Verification items for this drawing (mm, ordinates from the low corner). Give positions to 0.01 mm unless a question says otherwise; leave off trailing zeros. Order: outer loops, then holes, each group sorted by start corner. A loop starts at its lowest first (then second) coordinate and runs counter-clockwise, first axis right, second up. Notation, with made-up numbers: (11.25, -29) -> (33.25, -29) arc R17 ccw to (33.25, -13) -> close; hole circle Ø10 at (84.25, -29). An arc over 180 degrees is marked (long way). One line per question, with ' | ' between items.
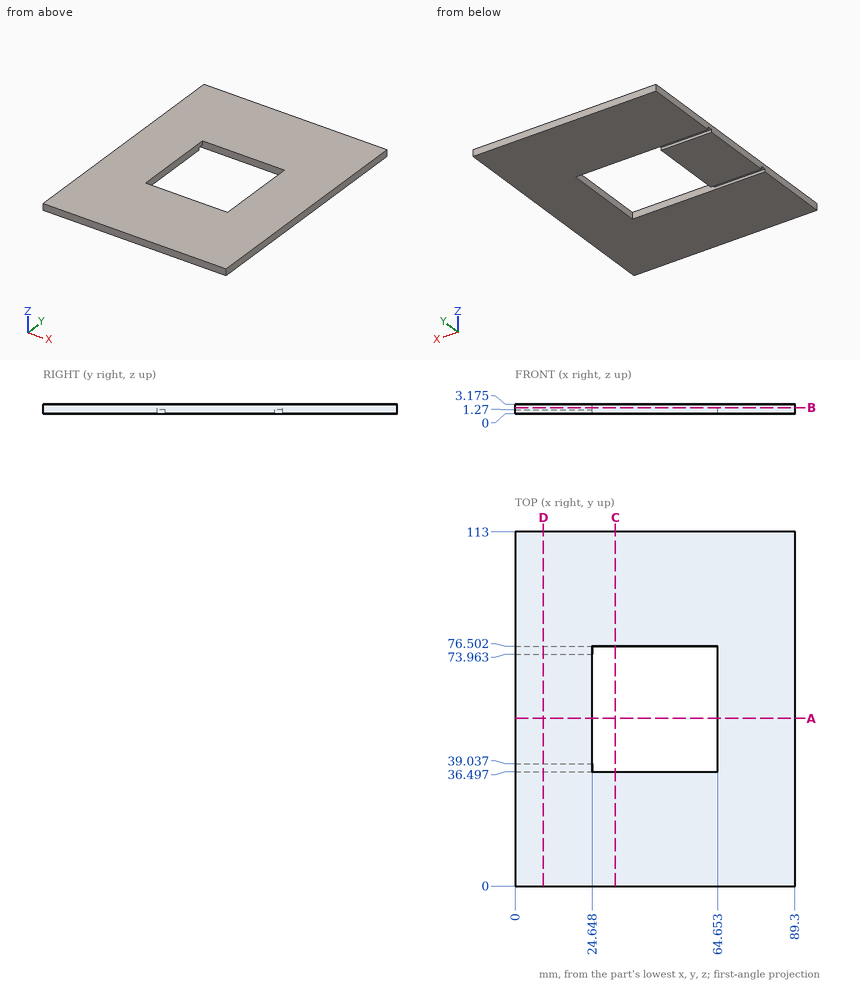
Q1. Section check C-C (x = 32). Enter the section's corners in (y, z) (1 decimal), and give its area (3 significant figures).
Result sheet:
outline: (0, 0) -> (36.5, 0) -> (36.5, 3.2) -> (0, 3.2) -> close; (76.5, 0) -> (113, 0) -> (113, 3.2) -> (76.5, 3.2) -> close | area: 232 mm2
Q2. Section check B-B (z = 2.05). Enter the section's corners in (x, y).
Result sheet:
outline: (0, 0) -> (89.3, 0) -> (89.3, 113) -> (0, 113) -> close; hole (24.65, 36.5) -> (64.65, 36.5) -> (64.65, 76.5) -> (24.65, 76.5) -> close
Q3. Thickness scan on line 1 (Y direction, x = 13.5, z = 0.8); line 2 (Y direction, x = 34, z = 0.9); line 3 (X direction, y = 60, z = 0.65). Record the ranges inside material, lowest first.
Result sheet:
line 1: y = 0 to 36.5, 39.04 to 73.96, 76.5 to 113 | line 2: y = 0 to 36.5, 76.5 to 113 | line 3: x = 0 to 24.65, 64.65 to 89.3
Q4. Depth check by flat-ended pin: pin 1 Ø1.3 at (x, y) = (15, 75) entering from -Z. Enter the tip coordinate at first touch or a pass-through.
Result sheet:
pin 1: stops at z = 1.27
Q5. Section check D-D (x = 9). Enter the section's corners in (y, z) (1 decimal).
Result sheet:
outline: (0, 0) -> (36.5, 0) -> (36.5, 1.3) -> (39, 1.3) -> (39, 0) -> (74, 0) -> (74, 1.3) -> (76.5, 1.3) -> (76.5, 0) -> (113, 0) -> (113, 3.2) -> (0, 3.2) -> close
Q6. Section check A-A (y = 53.5). Enter the section's corners in (x, z) (1 decimal).
Result sheet:
outline: (0, 0) -> (24.6, 0) -> (24.6, 3.2) -> (0, 3.2) -> close; (64.7, 0) -> (89.3, 0) -> (89.3, 3.2) -> (64.7, 3.2) -> close
